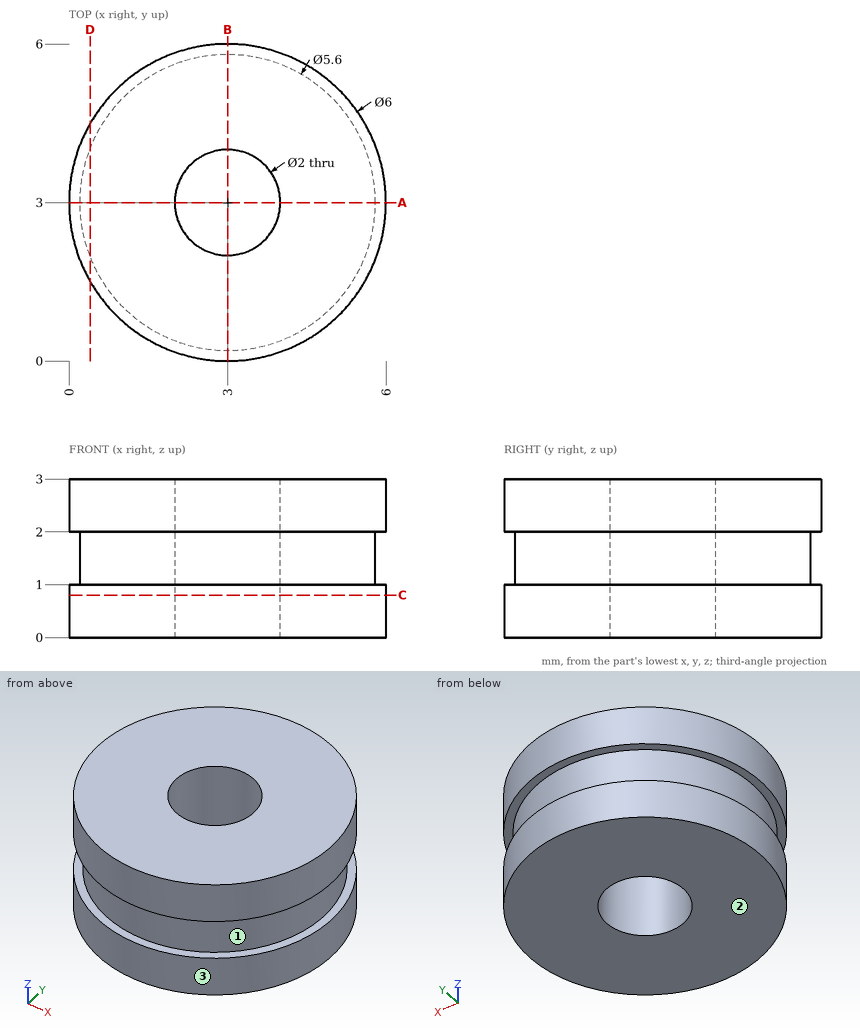
Design review of the part shown in the three views and the two pictorial views. Dimensions are in mm from the part's minimum x, y and z. Round coordinates to 2 decimals unless told otherwise and drop trailing zeros. Order: outer loops, then holes, each group sorted by start corner. A loop starts at its lowest first (then second) coordinate and runs counter-clockwise, first axis right, second up.
(1) Mouldability with a two-part tool opening along Z and no side actions: class the marked faces 1, 2 and 3 as released by +Z, released by -Z, zero draft, split by the parting line, or undercut.
Working result:
face 1: undercut
face 2: released by -Z
face 3: zero draft
(2) Wall thickness on L1, parallel to Y at x = 2.95, z = 0.2; L2, parallel to Y at x = 2.1, z = 2.65; L3, parallel to Y at x = 0.8, z = 1.3: over which ranges is each line inside the solid? List them lowest first.
Working result:
L1: y = 0 to 2, 4 to 6
L2: y = 0.14 to 2.56, 3.44 to 5.86
L3: y = 1.27 to 4.73
(3) Take a section at C-C, the plane z = 0.8. State the section outline as (x, y) points, plus the area to 3 significant figures.
Working result:
outline: circle Ø6 at (3, 3); hole circle Ø2 at (3, 3)
area: 25.1 mm2
(4) Take a section at A-A, the plane y = 3. State the section outline as (x, z) points.
Working result:
outline: (0, 0) - (2, 0) - (2, 3) - (0, 3) - (0, 2) - (0.2, 2) - (0.2, 1) - (0, 1) - close; (4, 0) - (6, 0) - (6, 1) - (5.8, 1) - (5.8, 2) - (6, 2) - (6, 3) - (4, 3) - close
(5) For P1, Ø1.5, axis at x = 4, z = 1, coming from the -Y side; P2, Ø1, axis at x = 5, z = 2, coming from the +Y side, all flat-tipped, find the tip position at first contact; note any pin that passes through.
Working result:
P1: stops at y = 0.01
P2: stops at y = 5.6
(6) Take a section at D-D, the plane x = 0.4. State the section outline as (y, z) points.
Working result:
outline: (1.5, 0) - (4.5, 0) - (4.5, 1) - (4.04, 1) - (4.04, 2) - (4.5, 2) - (4.5, 3) - (1.5, 3) - (1.5, 2) - (1.96, 2) - (1.96, 1) - (1.5, 1) - close
